Could you check a few things on this model? Use its own coordinates, in mm. A direction names the side the tool comes from. Give positions to 0.01 mm unless a question says otherwise; leave off trailing zeros. Loops run counter-clockwise (first coordinate to the right, second up) from the corner with the lowest first, then second, coordinate; pieces in that order, holes last. Notation, with made-up numbers: (-16, -40) - (-1, -40) arc R11 cw to (-1, -26) - close; hole circle Ø7 at (68.5, 78.5). An arc over 180 degrees is marked (long way). Answer in a Markdown table with one row per item. Add a question column.
```python
from build123d import *

# Parameters (mm, degrees)
SKETCH1_W           = 43
SKETCH1_H           = 11.5
SKETCH1_W_2         = 39
SKETCH1_H_2         = 7.5
BOSS_EXTRUDE1_DEPTH = 25
SKETCH2_W           = 43
SKETCH2_H           = 5.5
BOSS_EXTRUDE2_DEPTH = 4
SKETCH3_W           = 43
SKETCH3_H           = 2
BOSS_EXTRUDE3_DEPTH = 21


with BuildPart() as part:
    # Sketch1 → Boss-Extrude1 (new body)
    with BuildSketch(Plane(origin=(0, 0, 0), x_dir=(1, 0, 0), z_dir=(0, 1, 0))):
        with Locations((19.5, 3.75)):
            Rectangle(SKETCH1_W, SKETCH1_H)
        with Locations((19.5, 3.75)):
            Rectangle(SKETCH1_W_2, SKETCH1_H_2, mode=Mode.SUBTRACT)
    extrude(amount=BOSS_EXTRUDE1_DEPTH)

    # Sketch2 → Boss-Extrude2 (add)
    with BuildSketch(Plane.XZ):
        with Locations((19.5, 4.75)):
            Rectangle(SKETCH2_W, SKETCH2_H)
    extrude(amount=-BOSS_EXTRUDE2_DEPTH)

    # Sketch3 → Boss-Extrude3 (add)
    with BuildSketch(Plane(origin=(0, 4, 0), x_dir=(1, 0, 0), z_dir=(0, 1, 0))):
        with Locations((19.5, -6.5)):
            Rectangle(SKETCH3_W, SKETCH3_H)
    extrude(amount=BOSS_EXTRUDE3_DEPTH)


solid = part.part
```
(1) I want a section at B-B on x = 27. Please give me the cut outline in (y, z).
(2) On a 3-axis mill with a long thin cutter (end or side, diameter ignored), from which of +Z, -Z, +X, -X, +Y, -Y can I reach the whole of each face in a straight line? I mean faces 1 (the flat face through (41, 12, -3)), 2 (the flat face through (19, 4, 4)), 3 (the flat face through (0, 12, -4)). Say none if no direction works.
(3) I want a section at A-A on y = 20.75. Please give me the cut outline in (x, z), then the cut area to 3 significant figures.
(4) I want a section at D-D on z = 3.75. Please give me the cut outline in (x, y), then the cut area to 3 significant figures.
(5) We'd pull the mould along Z, two halves only. Please class faces 4 (the flat face through (19, 12, -9.5)), 5 (the flat face through (-2, 12, -3)), 6 (the flat face through (19, 12, -7.5)), 7 (the flat face through (19, 12, 7.5)): pulls with the +Z half, pulls with the -Z half, needs draft (parallel to the pull), parting line crosses it, or undercut.
(6) Please list where these lines run through material, in increasing order: line 1 (Z direction, x = 19, y = 21.5); line 2 (X direction, y = 9, z = -0.5); line 3 (Z direction, x = 22.5, y = 1.5).
(7) I want a section at C-C on z = -3. Please give me the cut outline in (x, y), then the cut area to 3 significant figures.
(8) For pin 1 Ø1.8 at (x, z) = (24, 3.5) entering from +Y, with a flat end and sliding along its axis, tell me the tip position at first contact or that it passes through.
Reported:
| question | item | result |
|---|---|---|
| 1 | outline | (0, -9.5) - (25, -9.5) - (25, -7.5) - (0, -7.5) - close; (0, 0) - (25, 0) - (25, 2) - (4, 2) - (4, 5.5) - (25, 5.5) - (25, 7.5) - (0, 7.5) - close |
| 2 | face 1 | +Z, -Z, +X, +Y, -Y |
| 2 | face 2 | +X, -X, +Y |
| 2 | face 3 | +Y, -Y |
| 3 | outline | (-2, -9.5) - (41, -9.5) - (41, 2) - (-2, 2) - close; (-2, 5.5) - (41, 5.5) - (41, 7.5) - (-2, 7.5) - close; hole (0, -7.5) - (39, -7.5) - (39, 0) - (0, 0) - close |
| 3 | area | 288 mm² |
| 4 | outline | (-2, 0) - (41, 0) - (41, 4) - (-2, 4) - close |
| 4 | area | 172 mm² |
| 5 | face 4 | pulls with the -Z half |
| 5 | face 5 | needs draft |
| 5 | face 6 | undercut |
| 5 | face 7 | pulls with the +Z half |
| 6 | line 1 | -9.5 to -7.5, 0 to 2, 5.5 to 7.5 |
| 6 | line 2 | -2 to 0, 39 to 41 |
| 6 | line 3 | -9.5 to -7.5, 0 to 7.5 |
| 7 | outline | (-2, 0) - (0, 0) - (0, 25) - (-2, 25) - close; (39, 0) - (41, 0) - (41, 25) - (39, 25) - close |
| 7 | area | 100 mm² |
| 8 | pin 1 | y = 4 |
